Solid Edge part; units mm, degrees
sketch "Sketch1" plane through (0, 0, 0) normal (0, -1, 0) x (1, 0, 0)
  line L0 (-5.3694, 18.9) -> (-19.0694, -4.8291)
  arc A0 (-13.7, -14.1291) -> (-19.0694, -4.8291) centre (-13.7, -7.9291) cw
  line L1 (-13.7, -14.1291) -> (13.7, -14.1291)
  arc A1 (19.0694, -4.8291) -> (13.7, -14.1291) centre (13.7, -7.9291) cw
  line L2 (5.3694, 18.9) -> (19.0694, -4.8291)
  arc A2 (-5.3694, 18.9) -> (5.3694, 18.9) centre (0, 15.8) cw
  dimension "D1" = 5.3694
extrude "Protrusion1" add sketch "Sketch1" against normal blind 14
sketch "Sketch2" plane through (0, 0, 0) normal (0, -1, 0) x (1, 0, 0)
  circle A0 centre (-13.7, -7.9291) radius 2.2
  circle A1 centre (13.7, -7.9291) radius 2.2
  circle A2 centre (0, 15.8) radius 2.2
extrude "Cutout1" cut sketch "Sketch2" against normal blind 457.8755
sketch "Sketch3" plane through (0, 0, 0) normal (0, -1, 0) x (1, 0, 0)
  circle A0 centre (0, 0) radius 5
extrude "Cutout2" cut sketch "Sketch3" against normal blind 434.4917
sketch "Sketch4" plane through (0, 0, 3.9355) normal (0, -1, 0) x (-0.5, 0, 0.8660254)
  line L0 (-23.325, -5.9323) -> (-23.325, -18.9323)
  line L1 (-23.325, -18.9323) -> (16.475, -18.9323)
  line L2 (16.475, -18.9323) -> (16.475, -5.9323)
  line L3 (12.7755, -8.7037) -> (16.475, -5.9323)
  line L4 (-20.9306, -8.7037) -> (12.7755, -8.7037)
  line L5 (-20.9306, -5.9323) -> (-20.9306, -8.7037)
  line L6 (-23.325, -5.9323) -> (-20.9306, -5.9323)
  dimension "D1" = 23.325
extrude "Protrusion2" add sketch "Sketch4" against normal up to vertex (14 mm away)
sketch "Sketch5" plane through (18.1083, 8, 10.4355) normal (0.8660254, 0, 0.5) x (-0.5, 0, 0.8660254)
  line L0 (-19.9, 8) -> (19.9, 8)
  line L1 (19.9, -6) -> (19.9, 8)
  line L2 (-19.9, -6) -> (19.9, -6)
  line L3 (-19.9, -6) -> (-19.9, 8)
extrude "ExtrudedProtrusion_14" add sketch "Sketch5" along normal blind 4
sketch "Sketch6" plane through (5.8112, 14, 7.7701) normal (0, 1, 0) x (0.5, 0, -0.8660254)
  circle A0 centre (3.8403, 24.7468) radius 3.7
  circle A1 centre (17.5403, 1.0177) radius 3.7
  circle A2 centre (-9.8597, 1.0177) radius 3.7
extrude "Cutout3" cut sketch "Sketch6" against normal blind 8
sketch "Sketch7" plane through (11.8615, 14, 7.7701) normal (0, 1, 0) x (-0.8660254, 0, -0.5)
  circle A0 centre (-2.5426, -0.8152) radius 2.2
extrude "ExtrudedCutout_23" cut sketch "Sketch7" against normal blind 166.5817
sketch "Sketch8" plane through (11.8615, 14, 7.7701) normal (0, 1, 0) x (-0.8660254, 0, -0.5)
  circle A0 centre (40.6865, -0.8152) radius 2.2
  line L0 (40.6865, 5.6848) -> (31.1282, 5.6848)
  line L1 (31.1282, 5.6848) -> (31.1282, 3.8832)
  line L2 (31.1282, 3.8832) -> (34.2429, 1.8592)
  line L3 (34.2429, 1.8592) -> (34.2429, -2.6486)
  line L4 (31.1282, -7.3152) -> (34.2429, -2.6486)
  line L5 (40.6865, -7.3152) -> (31.1282, -7.3152)
  arc A1 (40.6865, -7.3152) -> (40.6865, 5.6848) centre (40.6865, -0.8152) ccw
extrude "Protrusion3" add sketch "Sketch8" against normal up to vertex (14 mm away)
sketch "Sketch9" plane through (11.8615, 14, 7.7701) normal (0, 1, 0) x (-0.8660254, 0, -0.5)
  line L0 (-10.7426, -0.8152) -> (-10.7426, -20.7152)
  line L1 (-10.7426, -20.7152) -> (6.2574, -20.7152)
  arc A0 (1.1563, -18.0392) -> (6.2574, -20.7152) centre (6.2574, -14.5152) ccw
  line L2 (1.1563, -18.0392) -> (-10.7426, -0.8152)
extrude "Cutout4" cut sketch "Sketch9" against normal blind 85.4791
sketch "Sketch10" plane through (6.8865, 14, 7.7701) normal (0, 1, 0) x (-0.8660254, 0, -0.5)
  line L0 (-15.0511, 16.5973) -> (-15.0511, -3.3027)
  line L1 (-3.1522, 13.9213) -> (-15.0511, -3.3027)
  arc A0 (1.9489, 16.5973) -> (-3.1522, 13.9213) centre (1.9489, 10.3973) ccw
  line L2 (1.9489, 16.5973) -> (-15.0511, 16.5973)
extrude "ExtrudedCutout_27" cut sketch "Sketch10" against normal blind 118.3722
fillet "Round_1" radius 6.6 1 edges at (21.5724, 7, 12.4355)
sketch "Sketch11" plane through (-4.1206, 14, 1.1105) normal (0, 1, 0) x (0.0808589, 0, 0.9967256)
  line L0 (7.0612, 8.2038) -> (0.2016, 12.9426)
  arc A0 (-8.6084, 0.1899) -> (0.2016, 12.9426) centre (-0.7736, 4.1968) cw
  line L1 (-8.6084, 0.1899) -> (-1.7489, -4.5489)
  arc A1 (-1.7489, -4.5489) -> (7.0612, 8.2038) centre (-0.7736, 4.1968) ccw
extrude "ExtrudedCutout_28" cut sketch "Sketch11" against normal blind 3
Here's how the part is built. I have some questions about the finished solid (model axes, mm). A direction names the side the tool comes from. Coordinates: 2 decimals unless noted, no trailing zeros. Loops run counter-clockwise (first coordinate to the right, second up) from the corner with the lowest first, then second, coordinate; pieces in that order, holes last. Notation, with made-up numbers: M 87,50.5 L 111,50.5 A23 cw 111,85.5 Z; hole C 19,35.25 d1. An arc over 180 degrees is marked long. One line per item, written item: value.
1. Imagine slicing it at B-B (z = 15.8). List the corners of the cut face in (x, y) for me, and give its area (3 significant figures).
Geometry says:
outline: M -7.16,0 L -2.2,0 L -2.2,6 L -3.7,6 L -3.7,14 L -7.16,14 Z; M 2.2,0 L 14.47,0 L 14.47,14 L 3.7,14 L 3.7,6 L 2.2,6 Z
area: 217 mm2
2. Imagine slicing it at A-A (x = 0). List the corners of the cut face in (y, z) for me, and give its area (3 significant figures).
Geometry says:
outline: M 0,-14.13 L 14,-14.13 L 14,-8.8 L 11,-8.8 L 11,-5 L 0,-5 Z; M 0,5 L 11,5 L 11,8.8 L 14,8.8 L 14,12.1 L 6,12.1 L 6,13.6 L 0,13.6 Z; M 0,18 L 6,18 L 6,19.5 L 14,19.5 L 14,22 L 0,22 Z
area: 257 mm2
3. Please list where these lines run through material, in increasing order: probe 1 along Z at (x, y) = (0, 4.5); probe 2 along Z at (x, y) = (14.5, 11.5); probe 3 along X at (y, z) = (10.75, -7).
Geometry says:
probe 1: z = -14.13 to -5, 5 to 13.6, 18 to 22
probe 2: z = -14.08 to -11.54, -4.32 to 6.14, 10.54 to 15.79
probe 3: x = -25.09 to -17.28, -10.12 to 10.12, 17.28 to 20
4. On a 3-axis mill with a long thin cutter (end or side, diameter ignored), from which of +Z, -Z, +X, -X, +Y, -Y can I reach the whole of each face in a straight line? I mean faces 1 (the cylindrical face through (13.13, 7.1, 6.59)), 2 (the flat face through (1, 7, -14.129)), 3 (the cylindrical face through (-1.99, 10.06, 18.92)). Say none if no direction works.
Geometry says:
face 1: +Y, -Y
face 2: -Z, +X, +Y, -Y
face 3: +Y
5. Thinking about a two-plate mould opening in X: for faces 4 (the flat face through (-11.566, 6.902, 8.167)), 5 (the flat face through (2, 0, 6)), 6 (the flat face through (-16.1, 6, -8)), 7 (the flat face through (9.951, 7.098, 17.945)), which applies, +X half, -X half, draft (parallel to the pull), parting line (faces both ways), or undercut?
Geometry says:
face 4: -X half
face 5: draft
face 6: undercut
face 7: +X half
6. Will these pins go through, and if not, where does the flat tip stop? pin 1 Ø3 at (x, y) = (-12.5, 10.5) entering from -Z; pin 2 Ø2 at (y, z) = (10.5, -11) entering from +X; pin 3 Ø6 at (x, z) = (14.5, -6.5) entering from +Y; pin 4 Ø3 at (x, y) = (-18.5, 9) entering from +Z.
Geometry says:
pin 1: stops at z = -15.61
pin 2: stops at x = 19.54
pin 3: stops at y = 14
pin 4: stops at z = -1.24
7. Imagine slicing it at D-D (x = -13.7). List the corners of the cut face in (y, z) for me.
Geometry says:
outline: M 0,-15.43 L 14,-15.43 L 14,-11.63 L 6,-11.63 L 6,-10.13 L 0,-10.13 Z; M 0,-5.73 L 6,-5.73 L 6,-4.23 L 14,-4.23 L 14,4.47 L 0,4.47 Z
